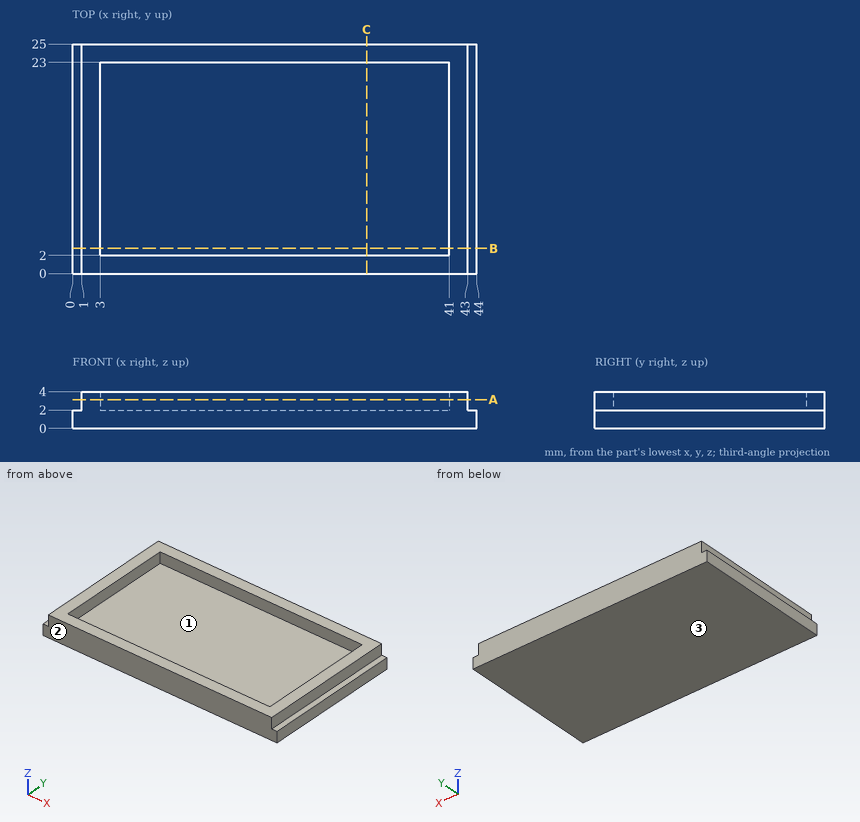
For this review, use the dimensioned drawing (mm, ordinates from the lowest corner) and the shaded views. Coordinates: 2 decimals unless noted, no trailing zeros. Loops run counter-clockwise (first coordinate to the right, second up) from the corner with the lowest first, then second, coordinate; pieces in that order, holes last. Notation, with made-up numbers: (81, -5) -> (139, -5) arc R17 cw to (139, 24) -> close; hole circle Ø2 at (-31, -2.75). An arc over 180 degrees is marked (long way). Write each question's results on one line, items separated by ' | '.
Q1. For pin 1 Ø1 at (x, z) = (20, 2.5) entering from -Y; pin 2 Ø0.6 at (y, z) = (15.5, 3) entering from +X; pin 3 Ø0.6 at (y, z) = (18, 3) entering from -X; pin 4 Ø1 at (x, y) = (18, 3) entering from +Z, all flat-tipped, find the tip position at first contact; note any pin that passes through.
Taken from the geometry:
pin 1: y = 0 | pin 2: x = 43 | pin 3: x = 1 | pin 4: z = 2
Q2. Add section A-A, the plane z = 3.15. State the section outline as (x, y) points.
Taken from the geometry:
outline: (1, 0) -> (43, 0) -> (43, 25) -> (1, 25) -> close; hole (3, 2) -> (41, 2) -> (41, 23) -> (3, 23) -> close
Q3. Add section C-C, the plane x = 32. State the section outline as (y, z) points.
Taken from the geometry:
outline: (0, 0) -> (25, 0) -> (25, 4) -> (23, 4) -> (23, 2) -> (2, 2) -> (2, 4) -> (0, 4) -> close
Q4. To check wall thickness, follow line 1 along X through (y, z) = (7.25, 2.5); line 2 along Y through (x, z) = (4.5, 2.3); line 3 along Z through (x, y) = (16, 21). State the ranges of each line that lie inside material, in increasing order. Write a range as [from, to].
Taken from the geometry:
line 1: [1, 3], [41, 43] | line 2: [0, 2], [23, 25] | line 3: [0, 2]
Q5. Add section B-B, the plane y = 2.75. State the section outline as (x, z) points, then the cut area to 3 significant figures.
Taken from the geometry:
outline: (0, 0) -> (44, 0) -> (44, 2) -> (43, 2) -> (43, 4) -> (41, 4) -> (41, 2) -> (3, 2) -> (3, 4) -> (1, 4) -> (1, 2) -> (0, 2) -> close | area: 96.0 mm²
Q6. Mouldability with a two-part tool opening along Y and no side actions: class the marked faces 1, 2 and 3 as +Y half, -Y half, draft (parallel to the pull), parting line (faces both ways), or undercut.
Taken from the geometry:
face 1: undercut | face 2: -Y half | face 3: draft
